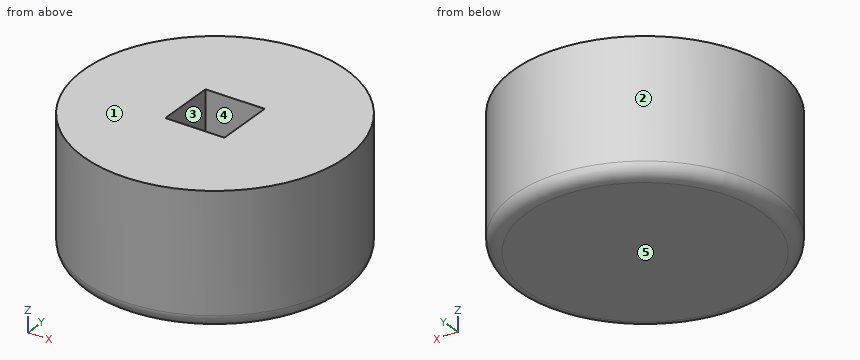
```python
from build123d import *

# Parameters (mm, degrees)
F0_R     = 20
F0_W     = 9
F0_H     = 9
F1_DEPTH = 3
F2_DEPTH = 20
F3_R     = 2


with BuildPart() as f1:
    # F0 (on Top) → F1 (new body)
    with BuildSketch(Plane.XY):
        Circle(F0_R)
        Rectangle(F0_W, F0_H, mode=Mode.SUBTRACT)
        Rectangle(F0_W, F0_H)
    extrude(amount=F1_DEPTH)

    # F0 (on Top) → F2 (join)
    with BuildSketch(Plane.XY):
        Circle(F0_R)
        Rectangle(F0_W, F0_H, mode=Mode.SUBTRACT)
    extrude(amount=F2_DEPTH)

    # F3
    f3_edges = [f1.edges().sort_by_distance(p)[0] for p in [
        (-20, 0, 0),
    ]]
    fillet(f3_edges, radius=F3_R)


solid = f1.part
```
Could you check a few things on this model? Use its own coordinates, in mm. Face numbers are marked on the shaded views. A direction names the side the tool comes from. Coordinates: 2 decimals unless noted, no trailing zeros. Order: outer loops, then holes, each group sorted by start corner. A loop starts at its lowest first (then second) coordinate and runs counter-clockwise, first axis right, second up. Notation, with made-up numbers: M 21,-17.75 L 35,-17.75 A16 cw 35,-1.75 Z; hole C -26,-39 d8. An arc over 180 degrees is marked long. Use a Markdown table: item, result. Add a question column.
Q1. I want a section at A-A on z = 3.5. List the corners of the cut face in (x, y) for me, then the cut area to 3 significant figures.
Q2. Which directions (+Z, -Z, +X, -X, +Y, -Y) give clear straight access to the entire face, cutting with the end or side of a thin tool? Please do the marked faces 4 and 5.
Q3. If I drill on L1, parallel to Y at x = 0, z = 18; L2, parallel to X at y = 3.5, z = 14.75; L3, parallel to Y at x = -1.5, z = 9.5, over which ranges is the centre line in solid material (lowest first)?
Q4. I'm going to push flat-ended pins straight in: pin 1 (4.5 mm diameter, centred on y = -2, z = 11.5, fed in from +X); pin 2 (2.5 mm diameter, centred on x = 1, y = -2, fed in from +Z); pin 3 (4 mm diameter, centred on y = 4, z = 3, fed in from -X); pin 4 (1 mm diameter, centred on x = -15.5, z = 6.5, fed in from +Y). Where does each tip first touch, or does it pass through?
Q5. I want a section at B-B on y = 0. List the corners of the cut face in (x, z) for me, then the cut area to 3 significant figures.
Q6. We'd pull the mould along Y, two halves only. Please class the marked faces 1, 2 and 3: pulls with the +Y half, pulls with the -Y half, needs draft (parallel to the pull), parting line crosses it, or undercut.
Checked values:
| question | item | result |
|---|---|---|
| 1 | outline | C 0,0 d40; hole M -4.5,-4.5 L 4.5,-4.5 L 4.5,4.5 L -4.5,4.5 Z |
| 1 | area | 1,180 mm² |
| 2 | face 4 | +Z |
| 2 | face 5 | -Z, +X, -X, +Y, -Y |
| 3 | L1 | -20 to -4.5, 4.5 to 20 |
| 3 | L2 | -19.69 to -4.5, 4.5 to 19.69 |
| 3 | L3 | -19.94 to -4.5, 4.5 to 19.94 |
| 4 | pin 1 | x = 20 |
| 4 | pin 2 | z = 3 |
| 4 | pin 3 | x = -19.9 |
| 4 | pin 4 | y = 13.23 |
| 5 | outline | M -20,2 A2 ccw -18,0 L 18,0 A2 ccw 20,2 L 20,20 L 4.5,20 L 4.5,3 L -4.5,3 L -4.5,20 L -20,20 Z |
| 5 | area | 645 mm² |
| 6 | face 1 | needs draft |
| 6 | face 2 | parting line crosses it |
| 6 | face 3 | undercut |
